from build123d import *

# Parameters (mm, degrees)
SKETCH1_R           = 1.5
BOSS_EXTRUDE1_DEPTH = 3
SKETCH3_W           = 4.615398666
SKETCH3_H           = 10
BOSS_EXTRUDE2_DEPTH = 12.9997796
FILLET7_R           = 1
CUT_EXTRUDE4_DEPTH  = 10
FILLET8_R           = 4
SKETCH8_W           = 76
SKETCH8_H           = 10
BOSS_EXTRUDE3_DEPTH = 4.615398666
SKETCH9_W           = 14.615398666
SKETCH9_H           = 12
SKETCH9_R           = 1.5
BOSS_EXTRUDE4_DEPTH = 3
FILLET9_R           = 5
FILLET10_R          = 5
SKETCH10_W          = 9.773230982
SKETCH10_H          = 9.985016007
SKETCH10_W_2        = 12.713773796
SKETCH10_H_2        = 7.76031956
CUT_EXTRUDE6_DEPTH  = 10
CUT_EXTRUDE7_DEPTH  = 46.992324429
BOSS_EXTRUDE5_DEPTH = 3


with BuildPart() as part:
    # Sketch1 → Boss-Extrude1 (new body)
    with BuildSketch(Plane(origin=(0, 0, 0), x_dir=(1, 0, 0), z_dir=(0, 1, 0))):
        Polygon((-3, -11.32792047), (3, -11.32792047), (3, -5), (7.615398666, -5), (7.615398666, 5), (3, 5), (3, 11.32792047), (-3, 11.32792047), align=None)
        with Locations(Location((0, 8.5, 0), (0, 0, 270))):
            Circle(SKETCH1_R, mode=Mode.SUBTRACT)
        with Locations(Location((0, -8.5, 0), (0, 0, 270))):
            Circle(SKETCH1_R, mode=Mode.SUBTRACT)
    extrude(amount=BOSS_EXTRUDE1_DEPTH)

    # Sketch3 → Boss-Extrude2 (add)
    with BuildSketch(Plane(origin=(0, 3, 0), x_dir=(1, 0, 0), z_dir=(0, 1, 0))):
        with Locations((5.307699333, 0)):
            Rectangle(SKETCH3_W, SKETCH3_H)
    extrude(amount=BOSS_EXTRUDE2_DEPTH)

    # Fillet7
    fillet7_edges = [part.edges().sort_by_distance(p)[0] for p in [
        (3, 1.5, 11.32792047),
        (3, 1.5, -11.32792047),
    ]]
    fillet(fillet7_edges, radius=FILLET7_R)

    # Sketch7 → Cut-Extrude4 (cut)
    with BuildSketch(Plane.XZ):
        with BuildLine():
            Line((-3.65526474, -6.392053518), (-3.78188192, 6.478485425))
            ThreePointArc((-3.78188192, 6.478485425), (-0.319780446, 0.076652438), (-3.65526474, -6.392053518))
        make_face()
    extrude(amount=-CUT_EXTRUDE4_DEPTH, mode=Mode.SUBTRACT)

    # Fillet8
    fillet8_edges = [part.edges().sort_by_distance(p)[0] for p in [
        (3, 3, 0),
    ]]
    fillet(fillet8_edges, radius=FILLET8_R)

    # Sketch8 → Boss-Extrude3 (add)
    with BuildSketch(Plane(origin=(7.615398666, 0, 0), x_dir=(0, 0, -1), z_dir=(1, 0, 0))):
        with Locations((0, 10.9997796)):
            Rectangle(SKETCH8_W, SKETCH8_H)
    extrude(amount=-BOSS_EXTRUDE3_DEPTH)

    # Sketch9 → Boss-Extrude4 (add)
    # profile 1 of 2: a face of its own
    with BuildSketch(Plane(origin=(0, 15.9997796, 0), x_dir=(1, 0, 0), z_dir=(0, 1, 0))):
        with Locations((10.307699333, 32)):
            Rectangle(SKETCH9_W, SKETCH9_H)
        with Locations(Location((12.745112207, 32.5, 0), (0, 0, 270))):
            Circle(SKETCH9_R, mode=Mode.SUBTRACT)
    # profile 2 of 2: a face of its own
    with BuildSketch(Plane(origin=(0, 15.9997796, 0), x_dir=(1, 0, 0), z_dir=(0, 1, 0))):
        with Locations((10.307699333, -32)):
            Rectangle(SKETCH9_W, SKETCH9_H)
        with Locations(Location((12.745112207, -32.5, 0), (0, 0, 270))):
            Circle(SKETCH9_R, mode=Mode.SUBTRACT)
    extrude(amount=BOSS_EXTRUDE4_DEPTH)

    # Fillet9
    # the kernel refuses this fillet: 5 mm, written as the material it adds along each edge
    with BuildSketch(Plane(origin=(7.615398666, 5.9997796, 5), x_dir=(0, -1, 0), z_dir=(-1, 0, 0))) as fillet9_piece_1:
        with BuildLine():
            CenterArc((FILLET9_R, FILLET9_R), FILLET9_R, 180, 90)
            Line((0, FILLET9_R), (0, 0))
            Line((0, 0), (FILLET9_R, 0))
        make_face()
    extrude(amount=4.615398666)

    # Fillet10
    # the kernel refuses this fillet: 5 mm, written as the material it adds along each edge
    with BuildSketch(Plane(origin=(3, 5.9997796, -5), x_dir=(0, -1, 0), z_dir=(1, 0, 0))) as fillet10_piece_1:
        with BuildLine():
            CenterArc((FILLET10_R, FILLET10_R), FILLET10_R, 180, 90)
            Line((0, FILLET10_R), (0, 0))
            Line((0, 0), (FILLET10_R, 0))
        make_face()
    extrude(amount=4.615398666)

    # Sketch10 → Cut-Extrude6 (cut)
    with BuildSketch(Plane(origin=(0, 3, 0), x_dir=(1, 0, 0), z_dir=(0, 1, 0))):
        with Locations((-1.330252474, 10.872508004)):
            Rectangle(SKETCH10_W, SKETCH10_H)
        with Locations((-2.800523881, -9.76015978)):
            Rectangle(SKETCH10_W_2, SKETCH10_H_2)
    extrude(amount=-CUT_EXTRUDE6_DEPTH, mode=Mode.SUBTRACT)

    # Sketch11 → Cut-Extrude7 (cut, through all)
    with BuildSketch(Plane(origin=(0, 18.9997796, 0), x_dir=(1, 0, 0), z_dir=(0, 1, 0))):
        with BuildLine():
            Line((14.245112207, 36), (14.245112207, 29))
            ThreePointArc((14.245112207, 29), (12.745112207, 27.5), (11.245112207, 29))
            Line((11.245112207, 29), (11.245112207, 36))
            ThreePointArc((11.245112207, 36), (12.745112207, 37.5), (14.245112207, 36))
        make_face()
        with BuildLine():
            Line((14.245112207, -29), (14.245112207, -36))
            ThreePointArc((14.245112207, -36), (12.745112207, -37.5), (11.245112207, -36))
            Line((11.245112207, -36), (11.245112207, -29))
            ThreePointArc((11.245112207, -29), (12.745112207, -27.5), (14.245112207, -29))
        make_face()
    extrude(amount=-CUT_EXTRUDE7_DEPTH, mode=Mode.SUBTRACT)

    # Sketch13 → Boss-Extrude5 (add)
    with BuildSketch(Plane(origin=(0, 18.9997796, 0), x_dir=(1, 0, 0), z_dir=(0, 1, 0))):
        Polygon((3, -38), (3, -39.5), (19.115398666, -39.5), (19.115398666, -24.5), (3, -24.5), (3, -26), (17.615398666, -26), (17.615398666, -38), align=None)
        Polygon((3, 26), (3, 24.5), (19.115398666, 24.5), (19.115398666, 39.5), (3, 39.5), (3, 38), (17.615398666, 38), (17.615398666, 26), align=None)
    extrude(amount=-BOSS_EXTRUDE5_DEPTH)


solid = part.part
Work out the finished part from the listing and answer in its coordinate system (mm). A direction names the side the tool comes from. Coordinates: 2 decimals unless noted, no trailing zeros. Loops run counter-clockwise (first coordinate to the right, second up) from the corner with the lowest first, then second, coordinate; pieces in that order, holes last. Notation, with made-up numbers: M -2,51.25 L 36,51.25 A20 cw 36,59.25 Z; hole C -23.5,48 d7. An arc over 180 degrees is marked long. Answer in a Markdown table with one row per item. Add a question column.
1. Consider L1, parallel to Z at x = 14.75, y = 17; L2, parallel to X at y = 18.25, z = 29; L3, parallel to Z at x = 6.25, y = 7. Determine where each line is inside the solid, lowest interval first.
2. Flat-ended cylindrical pins translate along their axes: P1, Ø1.4, axis at x = 5, z = 4.5, coming from the +Y side; P2, Ø4, axis at x = 0.5, y = 2, coming from the -Z side; P3, Ø7.5, axis at x = 7.5, z = -34, coming from the -Y side. Find the tip coordinate at first contact, or state that the pin passes through.
3. Find section C-C, the plane x = 6.75. Write down the section's boundary in (y, z).
4. Find section B-B, the plane z = 23. Write down the section's boundary in (x, y), then the cut area to 3 significant figures.
5. The mould has two halves that part along Z. Classify faces 4 (the flat face through (19.115, 18, 32)), 5 (the flat face through (2, 4, -5)), 6 (the cylindrical face through (12.7, 17.5, -37.5)), 7 (the flat face through (11, 18, -24.5)): pulls with the +Z half, pulls with the -Z half, needs draft (parallel to the pull), parting line crosses it, or undercut.
6. A tool of negligible diameter and unlimited length cuts with its end or side. For faces 1 (the flat face through (14.245, 18, 32)), 2 (the flat face through (5, 6, 24)), 3 (the flat face through (7.615, 10, -1)), from which of +Z, -Z, +X, -X, +Y, -Y can it reach the whole face along a straight path? Write none if from no direction.
7. Find section D-D, the plane y = 13.5. Write down the section's boundary in (x, z), then the cut area to 3 significant figures.
8. Find section A-A, the plane x = 16.5. Write down the section's boundary in (y, z), then the cut area to 3 significant figures.
Reported:
| question | item | result |
|---|---|---|
| 1 | L1 | z = -39.5 to -24.5, 24.5 to 39.5 |
| 1 | L2 | x = 3 to 11.25, 14.25 to 19.12 |
| 1 | L3 | z = -38 to 38 |
| 2 | P1 | stops at y = 16 |
| 2 | P2 | stops at z = -5.88 |
| 2 | P3 | stops at y = 6 |
| 3 | outline | M 0,-5 L 1,-5 A5 cw 6,-10 L 6,-38 L 16,-38 L 16,-39.5 L 19,-39.5 L 19,-24.5 L 16,-24.5 L 16,24.5 L 19,24.5 L 19,39.5 L 16,39.5 L 16,38 L 6,38 L 6,10 A5 cw 1,5 L 0,5 Z |
| 4 | outline | M 3,6 L 7.62,6 L 7.62,16 L 3,16 Z |
| 4 | area | 46.2 mm^2 |
| 5 | face 4 | needs draft |
| 5 | face 5 | pulls with the -Z half |
| 5 | face 6 | undercut |
| 5 | face 7 | undercut |
| 6 | face 1 | +Y, -Y |
| 6 | face 2 | +Z, +X, -X, -Y |
| 6 | face 3 | +Z, -Z, +X, -Y |
| 7 | outline | M 3,-38 L 7.62,-38 L 7.62,38 L 3,38 Z |
| 7 | area | 351 mm^2 |
| 8 | outline | M 16,-39.5 L 19,-39.5 L 19,-24.5 L 16,-24.5 Z; M 16,24.5 L 19,24.5 L 19,39.5 L 16,39.5 Z |
| 8 | area | 90.0 mm^2 |
